Here's how the part is built. I have some questions about the finished solid (model axes, mm). Face numbers are marked on the shaded views. Give positions to 0.01 mm unless a question says otherwise; leave off trailing zeros. One line per item, written item: value. Start each with the question number.
1) Please list where these lines run through material, in increasing order: L1, parallel to X at y = 19.5, z = -11.5; L2, parallel to Z at x = 0, y = 17 (3 decimals); L3, parallel to X at y = 10.5, z = 3. Write a range as [from, to].
2) Imagine slicing it at A-A on y = 10.75. Count the separate pieces of the cut face and the enclosed holes in it, plus the area to 3 significant figures.
3) We'd pull the mould along Z, two halves only. Please class the marked faces 1 and 2: +Z half, -Z half, draft (parallel to the pull), parting line (faces both ways), or undercut.
4) I'm going to push flat-ended pins straight in: P1, Ø6, axis at x = -20, y = 17.5, coming from the -Z side; P2, Ø8, axis at x = -11.51, z = 5.37, coming from the -Y side; P3, Ø8, axis at y = 11, z = 3.5, coming from the -X side. Where does each tip first touch, or does it pass through?
Autodesk Inventor part; units mm, degrees
ref_plane "Work Plane1" through (0, 21.59, 0) normal (0, 1, 0) x (1, 0, 0)
ref_plane "YZ Plane" through (0, 0, 0) normal (1, 0, 0) x (0, 1, 0)
ref_plane "XZ Plane" through (0, 0, 0) normal (0, 1, 0) x (-1, 0, 0)
sketch "Sketch6" plane through (0, 0, 0) normal (0, 0, 1) x (1, 0, 0)
  line L0 (540.6478, 1219.1491) -> (540.6478, -58.7076) construction
  line L1 (540.6478, -58.7076) -> (-407.4394, -58.7076) construction
  line L2 (-407.4394, -58.7076) -> (-407.4394, 1219.1491) construction
  line L3 (-407.4394, 1219.1491) -> (540.6478, 1219.1491) construction
  point P0 (0, 0)
sketch "Sketch5" plane through (0, 0, 0) normal (0, 0, 1) x (1, 0, 0)
  line L0 (0, 0) -> (0, 142.24)
  line L1 (0, 142.24) -> (50.8, 142.24)
  line L2 (50.8, 142.24) -> (-50.8, 142.24)
  line L3 (50.8, 142.24) -> (45.2986, 0) construction
  line L4 (45.2986, 0) -> (0, 0) construction
  spline S0 degree 2 poles (50.8, 142.24) (45.2986, 0) (0, 0) knots 1 1 1 2 2 2
  line L5 (-50.8, 142.24) -> (-45.2986, 0) construction
  line L6 (-45.2986, 0) -> (0, 0) construction
  spline S1 degree 2 poles (-50.8, 142.24) (-45.2986, 0) (0, 0) knots 1 1 1 2 2 2
  dimension "d20" = 142.24
  dimension "d21" = 50.8
  dimension "d22" = 101.6
revolve "Revolution1" add sketch "Sketch5" angle 360 about axis through (0, 0, 0) along (0, 1, 0) contours L0 L1 S0
ref_plane "Work Plane1" through (0, 21.59, 0) normal (0, 1, 0) x (1, 0, 0)
sketch "Sketch9" plane through (0, 21.59, 0) normal (0, 1, 0) x (1, 0, 0)
  line L0 (-101.4531, 67.0538) -> (104.6936, 67.0538)
  line L1 (104.6936, 67.0538) -> (104.6936, -70.5436)
  line L2 (104.6936, -70.5436) -> (-101.4531, -70.5436)
  line L3 (-101.4531, -70.5436) -> (-101.4531, 67.0538)
  point P0 (0, 0)
extrude "Extrusion2" cut sketch "Sketch9" along normal through all
sketch "Sketch10" plane through (0, 21.59, 0) normal (0, 1, 0) x (1, 0, 0)
  line L0 (0, 0) -> (0, 22.225)
  circle A0 centre (0, 22.225) radius 1.27
  circle A1 centre (-19.2474, 11.1125) radius 1.27
  circle A2 centre (-19.2474, -11.1125) radius 1.27
  circle A3 centre (0, -22.225) radius 1.27
  circle A4 centre (19.2474, -11.1125) radius 1.27
  circle A5 centre (19.2474, 11.1125) radius 1.27
  dimension "d75" = 22.225
  dimension "d76" = 2.54
  dimension "d79" = 360
extrude "Extrusion3" cut sketch "Sketch10" against normal blind 6.35
sketch "Sketch11" plane through (0, 21.59, 0) normal (0, 1, 0) x (1, 0, 0)
  line L0 (0, 0) -> (11.5101, -5.3673)
  line L1 (0, 0) -> (12.7, 0) construction
  line L2 (0, 0) -> (0, 4.6472)
  circle A0 centre (11.5101, -5.3673) radius 3
  circle A1 centre (-11.5101, -5.3673) radius 3
  dimension "d83" = 12.7
  dimension "d84" = 25
  dimension "d85" = 6
extrude "Extrusion4" cut sketch "Sketch11" against normal blind 25.4
properties part number "foreHullUpper" material "Polycarbonate, Clear"
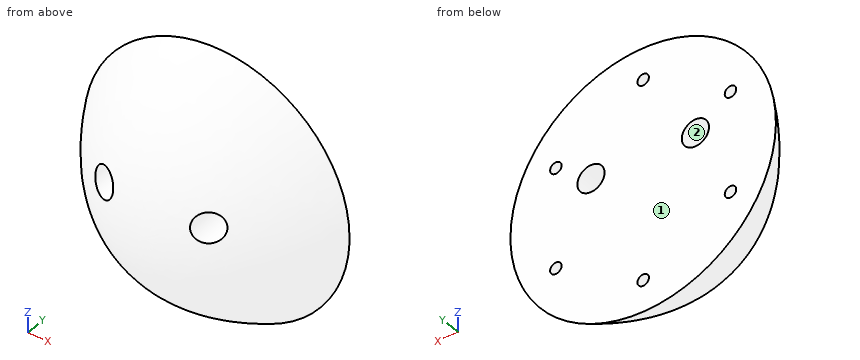
Numbers:
1. L1: [-25.63, -20.46], [-18.04, 18.04], [20.46, 25.63]
1. L2: [-26.564, -23.495], [-20.955, 20.955], [23.495, 26.564]
1. L3: [-21.47, -13.35], [-9.67, 9.67], [13.35, 21.47]
2. separate pieces: 1
2. enclosed holes: 2
2. area: 1,450 mm^2
3. face 1: draft
3. face 2: undercut
4. P1: z = -21.76
4. P2: y = 1.44
4. P3: x = -25.02
